from build123d import *

# Parameters (mm, degrees)
F0_R     = 56
F0_R_2   = 53
F1_DEPTH = 20
F2_R     = 56
F2_R_2   = 45.15
F3_DEPTH = 6.9
F4_R     = 56
F4_R_2   = 53
F5_DEPTH = 3
F6_R     = 62.5
F6_R_2   = 53
F7_DEPTH = 3


with BuildPart() as f1:
    # F0 (on Front) → F1 (new body)
    with BuildSketch(Plane.XZ):
        Circle(F0_R)
        Circle(F0_R_2, mode=Mode.SUBTRACT)
    extrude(amount=F1_DEPTH)

    # F2 (on face) → F3 (join)
    with BuildSketch(Plane.XZ.offset(20)):
        Circle(F2_R)
        Circle(F2_R_2, mode=Mode.SUBTRACT)
    extrude(amount=-F3_DEPTH)

    # F4 (on face) → F5 (join)
    with BuildSketch(Plane(origin=(0, 0, 0), x_dir=(-1, 0, 0), z_dir=(0, 1, 0))):
        Circle(F4_R)
        Circle(F4_R_2, mode=Mode.SUBTRACT)
    extrude(amount=F5_DEPTH)

    # F6 (on face) → F7 (join)
    with BuildSketch(Plane(origin=(0, 3, 0), x_dir=(-1, 0, 0), z_dir=(0, 1, 0))):
        Circle(F6_R)
        Circle(F6_R_2, mode=Mode.SUBTRACT)
    extrude(amount=F7_DEPTH)


solid = f1.part
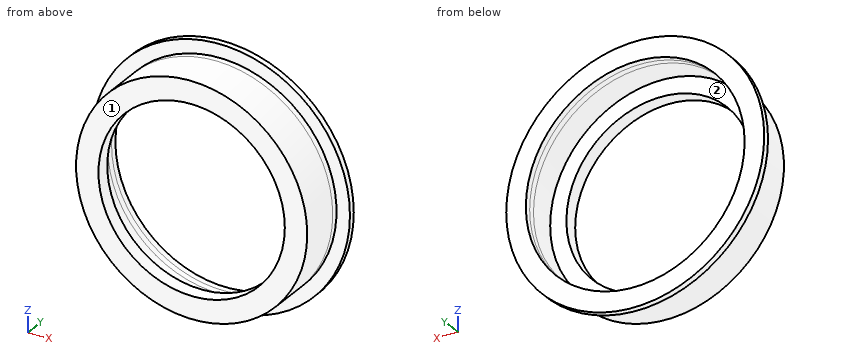
Check sheet for the modelled part. Datum: model origin and axes. Units: mm. Face numbers are marked on the shaded views. Give positions to 0.01 mm unless a question says otherwise; leave off trailing zeros. Order: outer loops, then holes, each group sorted by start corner. A loop starts at its lowest first (then second) coordinate and runs counter-clockwise, first axis right, second up. Notation, with made-up numbers: M 25,-3.75 L 71,-3.75 A22 cw 71,35.25 Z; hole C 26.5,-26.5 d1. An arc over 180 degrees is marked long. Answer as CSV lines item,"result". Start each with the question number.
Item 1: Gauge pin test, flat ends, axial feed: P1, Ø8, axis at y = -7.5, z = 10, coming from the -X side; P2, Ø2, axis at x = 47, z = 8, coming from the +Y side; P3, Ø1, axis at y = -17.5, z = -44.5, coming from the +X side. Record the tip position at first contact, or that the pin passes through.
Item 2: Mould release check, pull along X, two halves, no side actions. Record for the marked faces 1 and 2: +X half, -X half, draft (parallel to the pull), parting line (faces both ways), or undercut.
Item 3: Cross-section at C-C on y = -9. Enter the section's corners in (x, z).
Item 4: Thickness scan on line 1 (Z direction, x = 0, y = -16); line 2 (Z direction, x = 0, y = -8.75). Record the ranges inside material, lowest first. Write a range as [from, to].
Item 5: Cross-section at B-B on x = 0. Enter the section's corners in (y, z).
Item 6: Cross-section at A-A on z = 0. Enter the section's corners in (x, y), plus the area to 3 significant figures.
Item 7: Cross-section at D-D on x = -48. Enter the section's corners in (y, z), plus the area to 3 significant figures.
Established:
1,P1,"stops at x = -55.68"
1,P2,"stops at y = -13.1"
1,P3,"stops at x = 34.64"
2,face 1,"draft"
2,face 2,"undercut"
3,outline,"C 0,0 d112; hole C 0,0 d106"
4,line 1,"z = [-56, -45.15], [45.15, 56]"
4,line 2,"z = [-56, -53], [53, 56]"
5,outline,"M -20,-56 L 3,-56 L 3,-62.5 L 6,-62.5 L 6,-53 L -13.1,-53 L -13.1,-45.15 L -20,-45.15 Z; M -20,45.15 L -13.1,45.15 L -13.1,53 L 6,53 L 6,62.5 L 3,62.5 L 3,56 L -20,56 Z"
6,outline,"M -62.5,3 L -56,3 L -56,-20 L -45.15,-20 L -45.15,-13.1 L -53,-13.1 L -53,6 L -62.5,6 Z; M 45.15,-20 L 56,-20 L 56,3 L 62.5,3 L 62.5,6 L 53,6 L 53,-13.1 L 45.15,-13.1 Z"
6,area,"303 mm^2"
7,outline,"M -20,-28.84 L 3,-28.84 L 3,-40.03 L 6,-40.03 L 6,-22.47 L -13.1,-22.47 L -13.1,22.47 L 6,22.47 L 6,40.03 L 3,40.03 L 3,28.84 L -20,28.84 Z"
7,area,"709 mm^2"
